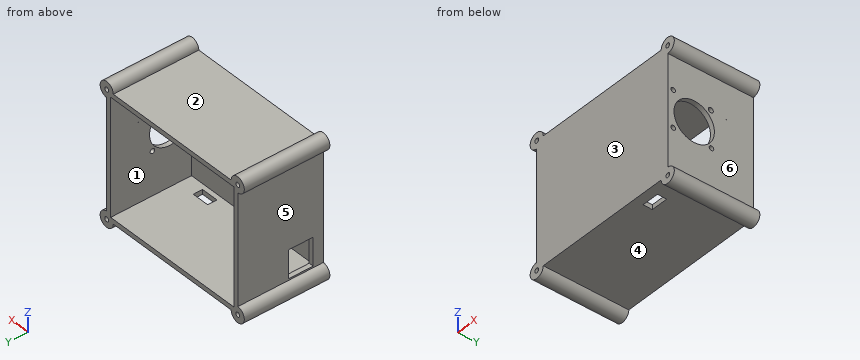
from build123d import *

# Parameters (mm, degrees)
SKETCH1_W           = 100
SKETCH1_H           = 80.8
BOSS_EXTRUDE1_DEPTH = 55
SKETCH2_W           = 94
SKETCH2_H           = 74.8
CUT_EXTRUDE1_DEPTH  = 52
SKETCH3_W           = 18
SKETCH3_H           = 16
CUT_EXTRUDE2_DEPTH  = 3
SKETCH4_W           = 11
SKETCH4_H           = 6
CUT_EXTRUDE3_DEPTH  = 3
SKETCH5_R           = 13
SKETCH5_W           = 0.144392858
SKETCH5_H           = 0.781479989
CUT_EXTRUDE5_DEPTH  = 3
SKETCH7_R           = 1.601751043
SKETCH7_R_2         = 1.47
CUT_EXTRUDE6_DEPTH  = 3
BOSS_EXTRUDE2_DEPTH = 55
BOSS_EXTRUDE3_DEPTH = 55
BOSS_EXTRUDE4_DEPTH = 55
BOSS_EXTRUDE5_DEPTH = 55
SKETCH13_R          = 1.47
CUT_EXTRUDE7_DEPTH  = 55
SKETCH14_R          = 1.47
CUT_EXTRUDE8_DEPTH  = 55
SKETCH15_R          = 1.47
CUT_EXTRUDE9_DEPTH  = 55
SKETCH16_R          = 1.47
CUT_EXTRUDE10_DEPTH = 55


with BuildPart() as part:
    # Sketch1 → Boss-Extrude1 (new body)
    with BuildSketch(Plane(origin=(0, 0, 0), x_dir=(1, 0, 0), z_dir=(0, 1, 0))):
        with Locations((-4.304593931, -21.292828061)):
            Rectangle(SKETCH1_W, SKETCH1_H)
    extrude(amount=BOSS_EXTRUDE1_DEPTH)

    # Sketch2 → Cut-Extrude1 (cut)
    with BuildSketch(Plane(origin=(0, 55, 0), x_dir=(1, 0, 0), z_dir=(0, 1, 0))):
        with Locations((-4.304593931, -21.292828061)):
            Rectangle(SKETCH2_W, SKETCH2_H)
    extrude(amount=-CUT_EXTRUDE1_DEPTH, mode=Mode.SUBTRACT)

    # Sketch3 → Cut-Extrude2 (cut)
    with BuildSketch(Plane.ZY.offset(54.304593931)):
        with Locations((-4.107171939, 14.5)):
            Rectangle(SKETCH3_W, SKETCH3_H)
    extrude(amount=-CUT_EXTRUDE2_DEPTH, mode=Mode.SUBTRACT)

    # Sketch4 → Cut-Extrude3 (cut)
    with BuildSketch(Plane(origin=(0, 0, -19.107171939), x_dir=(-1, 0, 0), z_dir=(0, 0, -1))):
        with Locations((-25.195406069, 9)):
            Rectangle(SKETCH4_W, SKETCH4_H)
    extrude(amount=-CUT_EXTRUDE3_DEPTH, mode=Mode.SUBTRACT)

    # Sketch5 → Cut-Extrude5 (cut)
    with BuildSketch(Plane(origin=(45.695406069, 0, 0), x_dir=(0, 0, -1), z_dir=(1, 0, 0))):
        with Locations((-22.692828061, 17)):
            Circle(SKETCH5_R)
        with Locations((-34.241433139, 37.409557734)):
            Rectangle(SKETCH5_W, SKETCH5_H)
    extrude(amount=-CUT_EXTRUDE5_DEPTH, mode=Mode.SUBTRACT)

    # Sketch7 → Cut-Extrude6 (cut)
    with BuildSketch(Plane(origin=(45.695406069, 0, 0), x_dir=(0, 0, -1), z_dir=(1, 0, 0))):
        with Locations((-35.2122597, 27.701622842)):
            Circle(SKETCH7_R)
        with Locations((-35.692828061, 3.5)):
            Circle(SKETCH7_R_2)
        with Locations((-12.192828061, 3.5)):
            Circle(SKETCH7_R_2)
        with Locations((-11.71600068, 28.120922326)):
            Circle(SKETCH7_R_2)
    extrude(amount=-CUT_EXTRUDE6_DEPTH, mode=Mode.SUBTRACT)

    # Sketch9 → Boss-Extrude2 (add)
    with BuildSketch(Plane(origin=(0, 55, 0), x_dir=(1, 0, 0), z_dir=(0, 1, 0))):
        with BuildLine():
            Line((41.695406069, 16.107171939), (42.695406069, 16.107171939))
            Line((42.695406069, 16.107171939), (42.695406069, 15.107171939))
            ThreePointArc((42.695406069, 15.107171939), (49.230939975, 22.642705845), (41.695406069, 16.107171939))
        make_face()
    extrude(amount=-BOSS_EXTRUDE2_DEPTH)

    # Sketch10 → Boss-Extrude3 (add)
    with BuildSketch(Plane(origin=(0, 55, 0), x_dir=(1, 0, 0), z_dir=(0, 1, 0))):
        with BuildLine():
            Line((-51.304593931, -57.692828061), (-51.304593931, -58.692828061))
            Line((-51.304593931, -58.692828061), (-50.304593931, -58.692828061))
            ThreePointArc((-50.304593931, -58.692828061), (-57.840127837, -65.228361967), (-51.304593931, -57.692828061))
        make_face()
    extrude(amount=-BOSS_EXTRUDE3_DEPTH)

    # Sketch11 → Boss-Extrude4 (add)
    with BuildSketch(Plane(origin=(0, 55, 0), x_dir=(1, 0, 0), z_dir=(0, 1, 0))):
        with BuildLine():
            Line((-50.304593931, 16.107171939), (-51.304593931, 16.107171939))
            Line((-51.304593931, 16.107171939), (-51.304593931, 15.107171939))
            ThreePointArc((-51.304593931, 15.107171939), (-57.840127837, 22.642705845), (-50.304593931, 16.107171939))
        make_face()
    extrude(amount=-BOSS_EXTRUDE4_DEPTH)

    # Sketch12 → Boss-Extrude5 (add)
    with BuildSketch(Plane(origin=(0, 55, 0), x_dir=(1, 0, 0), z_dir=(0, 1, 0))):
        with BuildLine():
            Line((41.695406069, -58.692828061), (42.695406069, -58.692828061))
            Line((42.695406069, -58.692828061), (42.695406069, -57.692828061))
            ThreePointArc((42.695406069, -57.692828061), (49.230939975, -65.228361967), (41.695406069, -58.692828061))
        make_face()
    extrude(amount=-BOSS_EXTRUDE5_DEPTH)

    # Sketch13 → Cut-Extrude7 (cut)
    with BuildSketch(Plane(origin=(0, 55, 0), x_dir=(1, 0, 0), z_dir=(0, 1, 0))):
        with Locations((45.695406069, -61.692828061)):
            Circle(SKETCH13_R)
    extrude(amount=-CUT_EXTRUDE7_DEPTH, mode=Mode.SUBTRACT)

    # Sketch14 → Cut-Extrude8 (cut)
    with BuildSketch(Plane(origin=(0, 55, 0), x_dir=(1, 0, 0), z_dir=(0, 1, 0))):
        with Locations((45.695406069, 19.107171939)):
            Circle(SKETCH14_R)
    extrude(amount=-CUT_EXTRUDE8_DEPTH, mode=Mode.SUBTRACT)

    # Sketch15 → Cut-Extrude9 (cut)
    with BuildSketch(Plane(origin=(0, 55, 0), x_dir=(1, 0, 0), z_dir=(0, 1, 0))):
        with Locations((-54.304593931, 19.107171939)):
            Circle(SKETCH15_R)
    extrude(amount=-CUT_EXTRUDE9_DEPTH, mode=Mode.SUBTRACT)

    # Sketch16 → Cut-Extrude10 (cut)
    with BuildSketch(Plane(origin=(0, 55, 0), x_dir=(1, 0, 0), z_dir=(0, 1, 0))):
        with Locations((-54.304593931, -61.692828061)):
            Circle(SKETCH16_R)
    extrude(amount=-CUT_EXTRUDE10_DEPTH, mode=Mode.SUBTRACT)


solid = part.part
For this review, take the finished solid that the model builds, in its own axes (mm). Face numbers are marked on the shaded views. A direction names the side the tool comes from. Round coordinates to 2 decimals unless told otherwise and drop trailing zeros. Order: outer loops, then holes, each group sorted by start corner. A loop starts at its lowest first (then second) coordinate and runs counter-clockwise, first axis right, second up. Notation, with made-up numbers: (72.5, 87) -> (100.5, 87) arc R27 ccw to (100.5, 103) -> close; hole circle Ø3 at (30.5, -30). An arc over 180 degrees is marked (long way). Put each result on its own line as item: value.
Q1. For probe 1 along Z at (x, y) = (18.5, 20.5); probe 2 along X at (y, z) = (40.5, -7.5); probe 3 along Z at (x, y) = (44.5, 7), list the stretches that pass through material, from the lowest coordinate up. Write a range as [from, to].
Check result:
probe 1: [-19.11, -16.11], [58.69, 61.69]
probe 2: [-54.3, -51.3], [42.7, 45.7]
probe 3: [-23.96, -19.96], [-18.25, 14.39], [31, 60.84], [62.55, 66.55]
Q2. Add section D-D on z = 24.5. Write out the cut boundary in (x, y).
Check result:
outline: (-54.3, 0) -> (45.7, 0) -> (45.7, 4.13) -> (42.7, 4.13) -> (42.7, 3) -> (-51.3, 3) -> (-51.3, 55) -> (-54.3, 55) -> close; (42.7, 29.87) -> (45.7, 29.87) -> (45.7, 55) -> (42.7, 55) -> close
Q3. Add section C-C on y = 33. Write out the cut boundary in (x, z), plus the area to 3 significant figures.
Check result:
outline: (-54.3, -14.11) arc R5 ccw (long way) to (-49.3, -19.11) -> (40.7, -19.11) arc R5 ccw (long way) to (45.7, -14.11) -> (45.7, 56.69) arc R5 ccw (long way) to (40.7, 61.69) -> (-49.3, 61.69) arc R5 ccw (long way) to (-54.3, 56.69) -> close; hole circle Ø2.94 at (-54.3, -19.11); hole circle Ø2.94 at (-54.3, 61.69); hole (-51.3, -16.11) -> (42.7, -16.11) -> (42.7, 58.69) -> (-51.3, 58.69) -> close; hole circle Ø2.94 at (45.7, -19.11); hole circle Ø2.94 at (45.7, 61.69)
area: 1,260 mm2
Q4. Machinability: for the marked faces 1, 2 and 3, which of the approach directions +Z, -Z, +X, -X, +Y, -Y give a long, thin tool a straight path to every point of the face, cutting with its end or side? Answer none if there is none.
Check result:
face 1: +Y
face 2: +Z, +Y, -Y
face 3: +Z, -Z, +X, -X, -Y
Q5. Mouldability with a two-part tool opening along X and no side actions: class the marked faces 4, 5 and 6 as pulls with the +X half, pulls with the -X half, needs draft (parallel to the pull), parting line crosses it, or undercut.
Check result:
face 4: undercut
face 5: pulls with the -X half
face 6: pulls with the +X half
Q6. Add section B-B on x = 36.5. Write out the cut boundary in (y, z).
Check result:
outline: (0, -19.11) -> (55, -19.11) -> (55, -16.11) -> (3, -16.11) -> (3, 58.69) -> (55, 58.69) -> (55, 61.69) -> (0, 61.69) -> close
Q7. Add section A-A on y = 17. Write out the cut boundary in (x, z).
Check result:
outline: (-54.3, -14.11) arc R5 ccw (long way) to (-49.3, -19.11) -> (40.7, -19.11) arc R5 ccw (long way) to (45.7, -14.11) -> (45.7, 9.69) -> (42.7, 9.69) -> (42.7, -16.11) -> (-51.3, -16.11) -> (-51.3, -13.11) -> (-54.3, -13.11) -> close; (-54.3, 4.89) -> (-51.3, 4.89) -> (-51.3, 58.69) -> (42.7, 58.69) -> (42.7, 35.69) -> (45.7, 35.69) -> (45.7, 56.69) arc R5 ccw (long way) to (40.7, 61.69) -> (-49.3, 61.69) arc R5 ccw (long way) to (-54.3, 56.69) -> close; hole circle Ø2.94 at (-54.3, -19.11); hole circle Ø2.94 at (-54.3, 61.69); hole circle Ø2.94 at (45.7, -19.11); hole circle Ø2.94 at (45.7, 61.69)
Q8. Insertion check: pin 1 Ø1.5 at (y, z) = (40.5, 50) entering from +X; pin 2 Ø4.5 at (y, z) = (3.5, 12.19) entering from -X; pin 3 Ø6 at (x, z) = (-10.5, -4.5) entering from +Y; pin 4 Ø2.5 at (x, z) = (-54.3, 61.69) entering from -Y. Each pin has a flat end and moves straight along its axis. Give the tip position at first contact, or say it passes through.
Check result:
pin 1: x = 45.7
pin 2: x = -54.3
pin 3: y = 3
pin 4: through
